Autodesk Inventor part; units mm, degrees
ref_plane "YZ Plane" through (0, 0, 0) normal (1, 0, 0) x (0, 1, 0)
ref_plane "XZ Plane" through (0, 0, 0) normal (0, 1, 0) x (-1, 0, 0)
ref_plane "XY Plane" through (0, 0, 0) normal (0, 0, 1) x (1, 0, 0)
sketch "Sketch1" plane through (0, 0, 0) normal (0, 1, 0) x (-1, 0, 0)
  circle A0 centre (0, 0) radius 1.115 construction
  arc A1 (-0.35, 1.3297) -> (-0.35, -1.3297) centre (0, 0) ccw
  circle A2 centre (0, 0) radius 4.5
  line L0 (0.35, 1.875) -> (-0.35, 1.875)
  line L1 (-0.35, 1.875) -> (-0.35, -1.875)
  line L2 (-0.35, -1.875) -> (0.35, -1.875)
  line L3 (0.35, -1.875) -> (0.35, 1.875)
  arc A3 (0.35, 1.3297) -> (-0.35, 1.3297) centre (0, 0) ccw
  arc A4 (0.35, -1.3297) -> (0.35, 1.3297) centre (0, 0) ccw
  arc A5 (-0.35, -1.3297) -> (0.35, -1.3297) centre (0, 0) ccw
  point P0 (0, 1.875)
  point P1 (0.35, 0)
  dimension "d1" = 2.23
  dimension "d3" = 9
  dimension "d18" = 0.26
  dimension "d19" = 0.7
  dimension "d20" = 3.75
extrude "Extrusion1" add sketch "Sketch1" along normal blind 3.5
sketch "Sketch4" plane through (0, 0, 0) normal (0, 0, 1) x (1, 0, 0)
  line L0 (-4.2, 17.5) -> (-4.2, 10.5)
  arc A0 (-4.2, 10.5) -> (4.2, 10.5) centre (0, 10.5) ccw
  line L1 (4.2, 10.5) -> (4.2, 17.5)
  line L2 (-3, 17.5) -> (-3, 14.8028)
  arc A1 (-3, 10.5) -> (3, 10.5) centre (0, 10.5) ccw
  line L3 (3, 10.5) -> (3, 11.1972)
  line L4 (-4.2, 17.5) -> (-3, 17.5)
  line L5 (3, 17.5) -> (4.2, 17.5)
  line L6 (-0.35, 0) -> (0.35, 0)
  line L7 (4.5, 3.5) -> (-4.5, 3.5)
  circle A2 centre (0, 13) radius 3.5
  line L8 (-3, 14.8028) -> (-3, 11.1972)
  line L9 (-3, 11.1972) -> (-3, 10.5)
  line L10 (3, 11.1972) -> (3, 14.8028)
  line L11 (3, 14.8028) -> (3, 17.5)
  point P0 (0, 0)
  point P1 (0, 0)
  dimension "d21" = 3
  dimension "d23" = 1.2
  dimension "d24" = 7
  dimension "d25" = 7
  dimension "d26" = 7
  dimension "d27" = 2.5
extrude "Extrusion5" add sketch "Sketch4" along normal mid plane 9 contours L4 L2 A2 L9 A1 L3 L11 L5 L1 A0 L0
sketch "Sketch8" plane through (0, 3.5, 0) normal (0, 1, 0) x (1, 0, 0)
  circle A0 centre (0, 0) radius 4
  arc A1 (0.35, -1.3297) -> (0.35, 1.3297) centre (0, 0) ccw
  line L0 (0.35, 1.875) -> (0.35, 1.3297)
  line L1 (-0.35, 1.875) -> (0.35, 1.875)
  line L2 (-0.35, 1.3297) -> (-0.35, 1.875)
  arc A2 (-0.35, 1.3297) -> (-0.35, -1.3297) centre (0, 0) ccw
  line L3 (-0.35, -1.875) -> (-0.35, -1.3297)
  line L4 (0.35, -1.875) -> (-0.35, -1.875)
  line L5 (0.35, -1.3297) -> (0.35, -1.875)
  dimension "d33" = 8
extrude "Extrusion6" add sketch "Sketch8" along normal up to next
sketch "Sketch2" plane through (0, 3.5, 0) normal (0, 1, 0) x (1, 0, 0)
  circle A0 centre (0, 0) radius 1.375
  circle A1 centre (0, 0) radius 3.375
  dimension "d6" = 2
  dimension "d9" = 7.3
  dimension "d10" = 2
properties part number "Laser Mount"
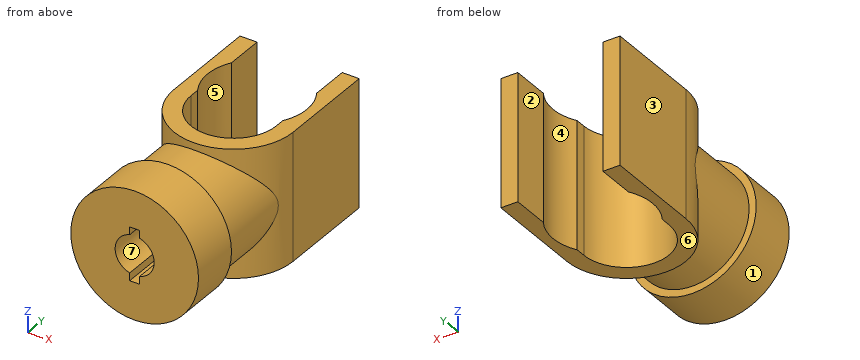
The listing builds one solid part. Answer for the finished solid, in the listing's coordinates (mm). Face numbers are marked on the shaded views. A direction names the side the tool comes from. Round coordinates to 2 decimals unless told otherwise and drop trailing zeros. Order: outer loops, then holes, each group sorted by start corner. A loop starts at its lowest first (then second) coordinate and runs counter-clockwise, first axis right, second up. Notation, with made-up numbers: M 11,45.25 L 26,45.25 A14 ccw 26,51.25 Z; hole C 47.25,47.5 d8. An arc over 180 degrees is marked long. Answer in a Markdown table with one row per item. Add a question column.
1) The part is cut by section B-B on y = 2.25. Determine the outline of the cut face in (x, z) (3 decimals).
2) The part is cut by section D-D on z = 0. Determine the outline of the cut face in (x, y) (3 decimals).
3) Which of the six approach directions +Z, -Z, +X, -X, +Y, -Y give full straight-line access (tool end or side, diameter ignored) to the marked faces 1, 2, 3 and 4?
4) Consider line 1 along X through (y, z) = (16, -1.75); line 2 along X through (y, z) = (9.75, -2); line 3 along Y through (x, z) = (2.5, -3.25). Determine where each line is inside the solid, lowest interval first. Write a range as from..to.
5) Flat-ended cylindrical pins translate along their axes: pin 1 Ø5 at (y, z) = (11, -1) entering from -X; pin 2 Ø1.3 at (y, z) = (15.5, 1.5) entering from +X; pin 3 Ø3 at (y, z) = (5.5, 2.5) entering from -X; pin 4 Ø1 at (x, z) = (-3.5, 2.5) entering from -Y. Find the tip coordinate at first contact, or state that the pin passes through.
6) The part is cut by section A-A on y = 15.25. Determine the outline of the cut face in (x, z), plus the area to 3 significant figures.
7) The part is cut by section C-C on x = 0. Determine the outline of the cut face in (y, z) (3 decimals).
8) Determine the mould class of the marked faces 5, 6 and 7 for opening direction Z: pulls with the +Z half, pulls with the -Z half, needs draft (parallel to the pull), parting line crosses it, or undercut.
Findings below:
| question | item | result |
|---|---|---|
| 1 | outline | C 0,0 d9; hole M -0.35,-1.875 L 0.35,-1.875 L 0.35,-1.33 A1.375 ccw 0.35,1.33 L 0.35,1.875 L -0.35,1.875 L -0.35,1.33 A1.375 ccw -0.35,-1.33 Z |
| 2 | outline | M -4.5,0 L -1.375,0 L -1.375,6.531 A4.2 ccw 1.375,6.531 L 1.375,0 L 4.5,0 L 4.5,3.5 L 4,3.5 L 4,9.219 A4.2 ccw 4.2,10.5 L 4.2,17.5 L 3,17.5 L 3,14.803 A3.5 cw 3,11.197 L 3,10.5 A3 cw -3,10.5 L -3,11.197 A3.5 cw -3,14.803 L -3,17.5 L -4.2,17.5 L -4.2,10.5 A4.2 ccw -4,9.219 L -4,3.5 L -4.5,3.5 Z |
| 3 | face 1 | -Y |
| 3 | face 2 | +Z, -Z, +Y |
| 3 | face 3 | +Z, -Z, -X, +Y |
| 3 | face 4 | +Z, -Z |
| 4 | line 1 | x = -4.2..-3, 3..4.2 |
| 4 | line 2 | x = -4.13..-2.9, 2.9..4.13 |
| 4 | line 3 | y = 0..3.5, 7.13..8.84 |
| 5 | pin 1 | stops at x = -4.2 |
| 5 | pin 2 | stops at x = 4.2 |
| 5 | pin 3 | stops at x = -3.87 |
| 5 | pin 4 | stops at y = 0 |
| 6 | outline | M -4.2,-4.5 L -3,-4.5 L -3,4.5 L -4.2,4.5 Z; M 3,-4.5 L 4.2,-4.5 L 4.2,4.5 L 3,4.5 Z |
| 6 | area | 21.6 mm² |
| 7 | outline | M 0,-4.5 L 3.5,-4.5 L 3.5,-4 L 6.3,-4 L 6.3,-4.5 L 7.5,-4.5 L 7.5,4.5 L 6.3,4.5 L 6.3,4 L 3.5,4 L 3.5,4.5 L 0,4.5 L 0,1.875 L 6.3,1.875 L 6.3,-1.875 L 0,-1.875 Z |
| 8 | face 5 | needs draft |
| 8 | face 6 | pulls with the -Z half |
| 8 | face 7 | undercut |
